For this review, use the dimensioned drawing (mm, ordinates from the lowest corner) and the shaded views. Coordinates: 2 decimals unless noted, no trailing zeros. Loops run counter-clockwise (first coordinate to the right, second up) from the corner with the lowest first, then second, coordinate; pieces in that order, holes last. Notation, with made-up numbers: (8.25, -3) - (64.25, -3) arc R17 cw to (64.25, 29) - close; hole circle Ø11 at (-2.5, 32.25). An arc over 180 degrees is marked (long way). Answer in a Markdown table with one row per item. Add a question column.
(1) We need section A-A, the plane x = 25. Write out the cut boundary in (y, z) (1 decimal), plus the area to 3 significant figures.
(2) We need section C-C, the plane z = 25. Write out the cut boundary in (x, y), plus the area to 3 significant figures.
(3) We need section D-D, the plane x = 34.5. Write out the cut boundary in (y, z).
(4) Clearance check with flat-ended pins moving along their axes: pin 1 (1.5 mm diameter, centred on x = 29.5, y = 8.5, fed in from +Z); pin 2 (5 mm diameter, centred on x = 28.5, y = 5, fed in from +Z) (1 decimal). State where each tip first meets the part, or that it passes through.
(5) We need section B-B, the plane y = 8.5. Write out the cut boundary in (x, z) (1 decimal).
(6) The part is to be moulded in two halves that separate along X. For the marked faces 1, 2, 3 and 4, say which applies: released by +X, released by -X, zero draft, split by the parting line, or undercut.
(7) To check wall thickness, follow L1, parallel to Z at x = 25, y = 3.5 (1 decimal); L2, parallel to X at y = 1, z = 24; L3, parallel to Z at x = 4, y = 9. State the ranges of each line that lie inside material, in increasing order. Write a range as [from, to].
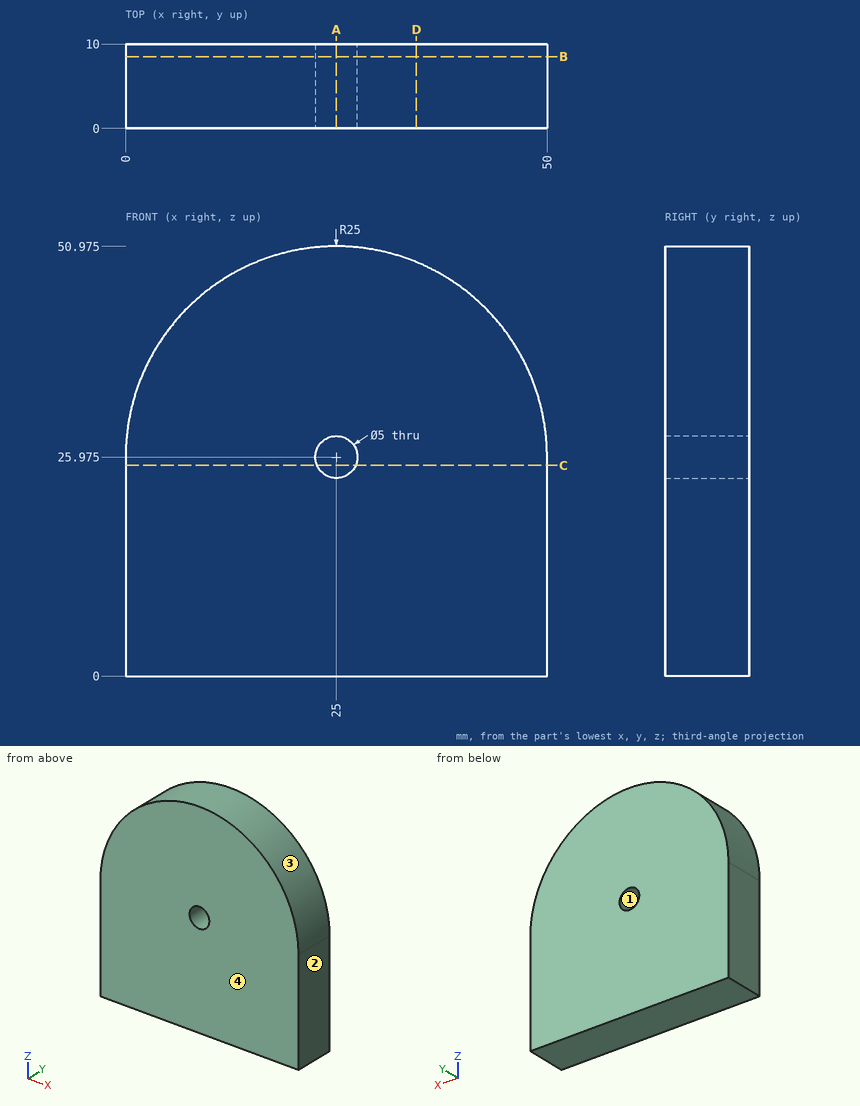
Responses:
| question | item | result |
|---|---|---|
| 1 | outline | (0, 0) - (10, 0) - (10, 23.5) - (0, 23.5) - close; (0, 28.5) - (10, 28.5) - (10, 51) - (0, 51) - close |
| 1 | area | 460 mm2 |
| 2 | outline | (0, 0) - (22.7, 0) - (22.7, 10) - (0, 10) - close; (27.3, 0) - (50, 0) - (50, 10) - (27.3, 10) - close |
| 2 | area | 454 mm2 |
| 3 | outline | (0, 0) - (10, 0) - (10, 49.1) - (0, 49.1) - close |
| 4 | pin 1 | stops at z = 50.69 |
| 4 | pin 2 | stops at z = 51 |
| 5 | outline | (0, 0) - (50, 0) - (50, 26) arc R25 ccw to (0, 26) - close; hole circle Ø5 at (25, 26) |
| 6 | face 1 | undercut |
| 6 | face 2 | released by +X |
| 6 | face 3 | split by the parting line |
| 6 | face 4 | zero draft |
| 7 | L1 | z = [0, 23.5], [28.5, 51] |
| 7 | L2 | x = [0, 23.47], [26.53, 50] |
| 7 | L3 | z = [0, 39.54] |
